```python
from build123d import *

# Parameters (mm, degrees)
SKETCH1_R           = 4
BOSS_EXTRUDE1_DEPTH = 9.525
SKETCH3_R           = 1.89865
SKETCH3_R_2         = 1.5875
CUT_EXTRUDE2_DEPTH  = 96.626232018
CUT_EXTRUDE6_DEPTH  = 96.626232018
FILLET1_R           = 2.54
CUT_EXTRUDE10_REACH = 169.521
SKETCH18_R          = 2.413
FILLET2_R           = 3.81


with BuildPart() as part:
    # Sketch1 → Boss-Extrude1 (new body)
    with BuildSketch(Plane.XY):
        with BuildLine():
            Line((-73.025, 20), (73.025, 20))
            Line((73.025, 20), (73.025, -20))
            Line((73.025, -20), (-73.025, -20))
            ThreePointArc((-73.025, -20), (-93.025, 0), (-73.025, 20))
        make_face()
        with Locations(Location((-73.025, 0, 0), (0, 0, 180))):
            Circle(SKETCH1_R, mode=Mode.SUBTRACT)
    extrude(amount=BOSS_EXTRUDE1_DEPTH)

    # Sketch3 → Cut-Extrude2 (cut, through all)
    with BuildSketch(Plane.XY):
        with Locations(Location((-73.025, 15, 0), (0, 0, 180))):
            Circle(SKETCH3_R)
        with Locations(Location((-58.025, 0, 0), (0, 0, 180))):
            Circle(SKETCH3_R)
        with Locations(Location((-73.025, -15, 0), (0, 0, 180))):
            Circle(SKETCH3_R)
        with Locations(Location((-88.025, 0, 0), (0, 0, 180))):
            Circle(SKETCH3_R)
        with Locations(Location((-83.631601718, 10.606601718, 0), (0, 0, 180))):
            Circle(SKETCH3_R_2)
        with Locations(Location((-62.418398282, 10.606601718, 0), (0, 0, 180))):
            Circle(SKETCH3_R_2)
        with Locations(Location((-62.418398282, -10.606601718, 0), (0, 0, 180))):
            Circle(SKETCH3_R_2)
        with Locations(Location((-83.631601718, -10.606601718, 0), (0, 0, 180))):
            Circle(SKETCH3_R_2)
    extrude(amount=CUT_EXTRUDE2_DEPTH, mode=Mode.SUBTRACT)

    # Sketch8 → Cut-Extrude6 (cut, through all)
    with BuildSketch(Plane.XY.offset(9.525)):
        Polygon((-50.501, 14), (-50.501, -14), (-10.738, -14), align=None)
        Polygon((-42.501, 14), (-2.738, -14), (-2.738, 14), align=None)
        Polygon((53.025, 14), (13.262, 14), (53.025, -14), (58.025, -14), (58.025, 14), align=None)
        Polygon((45.025, -14), (5.262, 14), (5.262, -14), align=None)
    extrude(amount=-CUT_EXTRUDE6_DEPTH, mode=Mode.SUBTRACT)

    # Fillet1
    fillet1_edges = [part.edges().sort_by_distance(p)[0] for p in [
        (58.025, -14, 4.7625),
        (53.025, -14, 4.7625),
        (13.262, 14, 4.7625),
        (58.025, 14, 4.7625),
        (5.262, -14, 4.7625),
        (5.262, 14, 4.7625),
        (45.025, -14, 4.7625),
        (-50.501, 14, 4.7625),
        (-10.738, -14, 4.7625),
        (-50.501, -14, 4.7625),
        (-2.738, 14, 4.7625),
        (-2.738, -14, 4.7625),
        (-42.501, 14, 4.7625),
    ]]
    fillet(fillet1_edges, radius=FILLET1_R)

    # Sketch18 → Cut-Extrude10 (cut, up to next)
    with BuildSketch(Plane(origin=(73.025, 0, 0), x_dir=(0, 0, -1), z_dir=(1, 0, 0)), mode=Mode.PRIVATE) as cut_extrude10_sk1:
        with Locations((-4.7625, 0)):
            Circle(SKETCH18_R)
    cut_extrude10_tool1 = extrude(cut_extrude10_sk1.sketch, amount=-CUT_EXTRUDE10_REACH, mode=Mode.PRIVATE) & part.part
    add(cut_extrude10_tool1.solids().sort_by_distance((73.025, 0, 4.7625))[0], mode=Mode.SUBTRACT)

    # Fillet2
    fillet2_edges = [part.edges().sort_by_distance(p)[0] for p in [
        (73.025, -20, 4.7625),
        (73.025, 20, 4.7625),
    ]]
    fillet(fillet2_edges, radius=FILLET2_R)


solid = part.part
```
Build history of the part. All positions in model axes, mm. A direction names the side the tool comes from. Give positions to 0.01 mm unless a question says otherwise; leave off trailing zeros. Loops run counter-clockwise (first coordinate to the right, second up) from the corner with the lowest first, then second, coordinate; pieces in that order, holes last. Notation, with made-up numbers: (-20.75, -12.5) - (37.25, -12.5) arc R15 cw to (37.25, -7.5) - close; hole circle Ø11 at (-19.75, -38). An arc over 180 degrees is marked (long way). Use a Markdown table: item, result.
(1) Band-saw the part on A-A (x = -44.5). Give the cut face in (y, z) (3 decimals), and give its area (3 significant figures).
Taken from the geometry:
| item | result |
|---|---|
| outline | (-20, 0) - (-14, 0) - (-14, 9.525) - (-20, 9.525) - close; (9.774, 0) - (20, 0) - (20, 9.525) - (9.774, 9.525) - close |
| area | 155 mm2 |
(2) Drop flat-ended pins along their axis: pin 1 Ø4 at (y, z) = (13, 7) entering from -X; pin 2 Ø3 at (y, z) = (-3.5, 6) entering from -X; pin 3 Ø3 at (x, y) = (30, -6.5) entering from +Z; pin 4 Ø1.5 at (y, z) = (15, 4.5) entering from -X. Give the stop position or say it passes through.
Taken from the geometry:
| item | result |
|---|---|
| pin 1 | x = -89.73 |
| pin 2 | x = -92.92 |
| pin 3 | through |
| pin 4 | x = -87.06 |
(3) Band-saw the part on B-B (z = 4). Give the number of separate pieces and of enclosed holes in the cut face, and give its area (3 significant figures).
Taken from the geometry:
| item | result |
|---|---|
| separate pieces | 1 |
| enclosed holes | 12 |
| area | 3,970 mm2 |
(4) Pull direction Y, two halves, no side cores. Call faces 3 (the face through (-27, 0, 0)), 4 (the face through (-49.17, 11.34, 4.7)), 5 (the face through (-3, 20, 5)): +Y half, -Y half, draft (parallel to the pull), parting line (faces both ways), or undercut.
Taken from the geometry:
| item | result |
|---|---|
| face 3 | draft |
| face 4 | undercut |
| face 5 | +Y half |
(5) Which spindle directions (+Z, -Z, +X, -X, +Y, -Y) get a long thin tool onto all of the face, cutting with end or side? Do faces 1 (the face through (73.025, 0, 8)), 2 (the face through (-31.692, 0.755, 4.829)). Say none if no direction does.
Taken from the geometry:
| item | result |
|---|---|
| face 1 | +Z, -Z, +X, +Y, -Y |
| face 2 | +Z, -Z |
(6) Wall check: line 1 along Y through (x, z) = (21, 8); line 2 along X through (y, z) = (2.5, 2) (1 decimal); line 3 along Y through (x, z) = (-20, 1.5). Give the ranges that are in metal, low to high.
Taken from the geometry:
| item | result |
|---|---|
| line 1 | -20 to -14, 2.92 to 8.55, 13.98 to 20 |
| line 2 | -92.9 to -76.1, -69.9 to -50.5, -34.2 to -26.2, -2.7 to 5.3, 21.6 to 29.6, 58 to 73 |
| line 3 | -20 to -14, -7.48 to -1.84, 14 to 20 |
